Autodesk Inventor part; units mm, degrees
ref_plane "YZ Plane" through (0, 0, 0) normal (1, 0, 0) x (0, 1, 0)
ref_plane "XZ Plane" through (0, 0, 0) normal (0, 1, 0) x (-1, 0, 0)
ref_plane "XY Plane" through (0, 0, 0) normal (0, 0, 1) x (1, 0, 0)
sketch "Sketch1" plane through (0, 0, 0) normal (0, 1, 0) x (-1, 0, 0)
  line L0 (-25, 25) -> (-25, -25)
  line L1 (-25, -25) -> (25, -25)
  line L2 (25, -25) -> (25, 25)
  line L3 (25, 25) -> (-25, 25)
  line L4 (-25, 25) -> (25, -25) construction
  line L5 (-25, -25) -> (25, 25) construction
  point P0 (0, 0)
  dimension "d0" = 50
  dimension "d1" = 50
extrude "Extrusion1" add sketch "Sketch1" along normal blind 1
sketch "Sketch2" plane through (0, 1, 0) normal (0, 1, 0) x (1, 0, 0)
  line L0 (25, -25) -> (25, 25) construction
  line L1 (25, -25) -> (25, -20) construction
  line L2 (25, -20) -> (-25, -20) construction
  line L3 (-25, 25) -> (-25, -25) construction
  line L4 (25, -20) -> (25, -2) construction
  line L5 (25, -2) -> (-25, -2) construction
  line L6 (25, -20) -> (18, -20) construction
  line L7 (18, -20) -> (18, -2) construction
  line L8 (-25, -20) -> (-18, -20) construction
  line L9 (-18, -20) -> (-18, -2) construction
  line L10 (1, -2) -> (-1, -2) construction
  line L11 (-1, -2) -> (-1, -20) construction
  line L12 (-1, -20) -> (1, -20) construction
  line L13 (1, -20) -> (1, -2) construction
  line L14 (1, -2) -> (-1, -20) construction
  line L15 (-1, -2) -> (1, -20) construction
  line L16 (18, -2) -> (1, -2)
  line L17 (1, -2) -> (1, -20)
  line L18 (1, -20) -> (18, -20)
  line L19 (18, -20) -> (18, -2)
  line L20 (-1, -2) -> (-18, -2)
  line L21 (-18, -2) -> (-18, -20)
  line L22 (-18, -20) -> (-1, -20)
  line L23 (-1, -20) -> (-1, -2)
  point P0 (0, 0)
  point P1 (0, -11)
  dimension "d4" = 5
  dimension "d5" = 18
  dimension "d6" = 7
  dimension "d7" = 7
  dimension "d8" = 2
extrude "Extrusion2" add sketch "Sketch2" along normal blind 15
sketch "Sketch3" plane through (0, 1, 0) normal (0, 1, 0) x (1, 0, 0)
  line L0 (18, -20) -> (1, -20)
  line L1 (18, -20) -> (18, -25)
  line L2 (-25, -25) -> (25, -25)
  line L3 (1, -20) -> (1, -25)
  line L4 (1, -25) -> (18, -25)
  line L5 (18, -20) -> (1, -20)
  line L6 (18, -25) -> (12.33, -25)
  line L7 (12.33, -25) -> (12.33, -20)
  line L8 (18, -20) -> (12.33, -20)
  line L9 (12.33, -20) -> (6.66, -20)
  line L10 (6.66, -20) -> (6.66, -25)
  line L11 (6.66, -20) -> (1, -20)
  point P0 (0, 0)
  dimension "d11" = 5.67
  dimension "d12" = 5.67
extrude "Extrusion3" add sketch "Sketch3" along normal blind 11
sketch "Sketch4" plane through (18, 1, 25) normal (1, 0, 0) x (0, 0, -1)
  line L0 (5, 11) -> (5, 15)
  line L1 (5, 11) -> (4, 11)
  line L2 (0, 11) -> (5, 11)
  line L3 (4, 11) -> (5, 9.2085)
  line L4 (5, 0) -> (5, 15)
  point P0 (25, -1)
  dimension "d9" = 15
  dimension "d15" = 1
extrude "Extrusion4" cut sketch "Sketch4" against normal through all
sketch "Sketch5" plane through (0, 12, 0) normal (0, 1, 0) x (1, 0, 0)
  line L0 (18, -25) -> (18, -21) construction
  line L1 (18, -21) -> (12.33, -21) construction
  line L2 (18, -21) -> (1, -21) construction
  line L3 (12.33, -21) -> (12.33, -25.0141) construction
  line L4 (12.33, -25.0141) -> (6.66, -25) construction
  line L5 (1, -25) -> (18, -25) construction
  line L6 (6.66, -25) -> (6.67, -21) construction
  line L7 (6.67, -21) -> (1, -21) construction
  line L8 (-25, -25) -> (1, -25) construction
  line L9 (1, -21) -> (1, -25) construction
  circle A0 centre (3.835, -23) radius 1.625
  circle A1 centre (9.5, -23) radius 1.625
  circle A2 centre (15.165, -23) radius 1.625
  point P0 (0, 0)
  dimension "d18" = 5.67
  dimension "d19" = 5.67
  dimension "d20" = 5.67
  dimension "d21" = 3.25
  dimension "d22" = 3.25
  dimension "d23" = 3.25
extrude "Extrusion5" cut sketch "Sketch5" against normal blind 1.5
sketch "Sketch6" plane through (-25, 0, 25) normal (0, 0, 1) x (1, 0, 0)
  line L0 (0, 1) -> (26, 1)
  line L1 (26, 1) -> (43.0101, 1)
  line L2 (26, 12) -> (43, 12) construction
  line L3 (26, 12) -> (31.67, 12) construction
  line L4 (31.67, 12) -> (31.67, 1) construction
  line L5 (31.67, 1) -> (37.34, 1) construction
  line L6 (50, 1) -> (0, 1) construction
  line L7 (37.34, 1) -> (37.34, 12) construction
  line L8 (26.835, 6.1045) -> (30.835, 6.1045)
  line L9 (30.835, 6.1045) -> (30.835, 2.1045)
  line L10 (30.835, 2.1045) -> (26.835, 2.1045)
  line L11 (26.835, 2.1045) -> (26.835, 6.1045)
  line L12 (26.835, 6.1045) -> (30.835, 2.1045) construction
  line L13 (30.835, 6.1045) -> (26.835, 2.1045) construction
  point P0 (25, 0)
  point P1 (28.835, 4.1045)
  dimension "d26" = 5.67
  dimension "d27" = 5.67
  dimension "d28" = 4
  dimension "d29" = 4
extrude "Extrusion6" cut sketch "Sketch6" against normal blind 2
ref_plane "Work Plane1" through (9.5, 1, 2) normal (-1, 0, 0) x (0, 0, 1)
mirror "Mirror1" about plane through (9.5, 1, 2) normal (-1, 0, 0) of "Extrusion6"
ref_plane "Work Plane2" through (6.6675, 1, 2) normal (-1, 0, 0) x (0, 0, 1)
mirror "Mirror2" about plane through (6.6675, 1, 2) normal (-1, 0, 0) of "Extrusion6"
ref_plane "Work Plane3" through (0, 0, -25) normal (-1, 0, 0) x (0, 0, 1)
mirror "Mirror3" about plane through (0, 0, -25) normal (-1, 0, 0) of "Extrusion3", "Extrusion5", "Extrusion6", "Mirror1", "Mirror2", "Extrusion2"
sketch "Sketch7" plane through (0, 1, 0) normal (0, 1, 0) x (1, 0, 0)
  line L0 (25, 25) -> (25, 23) construction
  line L1 (25, -25) -> (25, 25) construction
  line L2 (25, 23) -> (23, 23) construction
  line L3 (23, 23) -> (13, 23)
  line L4 (13, 23) -> (13, 20.4297)
  line L5 (13, 20.4297) -> (23, 20.4297)
  line L6 (23, 20.4297) -> (23, 23)
  line L7 (18, 20.4297) -> (18, 23)
  line L8 (18, 20.4297) -> (23, 20.4297)
  line L9 (20.5, 20.4297) -> (20.5, 23)
  line L10 (18, 20.4297) -> (13, 20.4297)
  line L11 (15.5, 20.4297) -> (15.5, 23)
  circle A0 centre (21.75, 21.6797) radius 1.25
  circle A1 centre (19.25, 21.6797) radius 1.25
  circle A2 centre (16.75, 21.6797) radius 1.25
  circle A3 centre (14.25, 21.6797) radius 1.25
  circle A4 centre (21.75, 21.6797) radius 0.75
  circle A5 centre (19.25, 21.6797) radius 0.75
  circle A6 centre (16.75, 21.6797) radius 0.75
  circle A7 centre (14.25, 21.6797) radius 0.75
  point P0 (0, 0)
  dimension "d33" = 2
  dimension "d34" = 2
  dimension "d35" = 10
  dimension "d36" = 0.5
  dimension "d37" = 0.5
  dimension "d38" = 0.5
  dimension "d39" = 0.5
extrude "Extrusion7" add sketch "Sketch7" along normal blind 5 contours A4 | A5 | A6 | A7
extrude "Extrusion8" add sketch "Sketch7" along normal blind 1 contours L6 A0 L9 L3 | L9 A1 L7 L3 | A0 | L6 L5 A0 | L7 A2 L11 L3 | A0 L5 L9 | A1 | L9 L5 A1 | L11 A3 L4 L3 | A1 L5 L7 | A2 | L7 L5 A2 | A2 L5 L11 | A3 | L11 L5 A3 | A3 L5 L4 | A4 | A5 | A6 | A7
properties part number "H Bridge #2"
Here's how the part is built. I have some questions about the finished solid (model axes, mm). A direction names the side the tool comes from. Give positions to 0.01 mm unless a question says otherwise; leave off trailing zeros. Loops run counter-clockwise (first coordinate to the right, second up) from the corner with the lowest first, then second, coordinate; pieces in that order, holes last. Notation, with made-up numbers: M 72.25,25.25 L 95.25,25.25 A27 cw 95.25,55.25 Z; hole C 24,65 d9. An arc over 180 degrees is marked long. Return JSON: item names as keys, results as strings.
Item 1: Thinking about a two-plate mould opening in X: for faces 4 (the flat face through (-10, 14, 20)), 5 (the flat face through (9, 6.104, 24)), which applies, released by +X, released by -X, zero draft, split by the parting line, or undercut?
A:
{"face 4": "zero draft", "face 5": "undercut"}
Item 2: On a 3-axis mill with a long thin cutter (end or side, diameter ignored), from which of +Z, -Z, +X, -X, +Y, -Y can I reach the whole of each face in a straight line? I mean faces 1 (the flat face through (22, 6, -22)), 2 (the flat face through (-13.165, 4, 24)), 3 (the cylindrical face through (21, 3.97, -21.65)). Say none if no direction works.
A:
{"face 1": "+Z, -Z, +X, -X, +Y", "face 2": "+Z", "face 3": "+Y"}
Item 3: Imagine slicing it at A-A on y = 9. List the corners of the cut face in (x, z) for me.
A:
{"outline": "M -18,2 L -1,2 L -1,25 L -18,25 Z; M 1,2 L 18,2 L 18,25 L 1,25 Z"}
Item 4: I'm going to push flat-ended pins straight in: pin 1 Ø1.5 at (y, z) = (11.5, -0.5) entering from -X; pin 2 Ø0.6 at (y, z) = (4.5, 24) entering from +X; pin 3 Ø1.9 at (x, z) = (-3.835, 23) entering from +Y; pin 4 Ø3.5 at (x, z) = (3.835, 23) entering from +Y. Where does each tip first touch, or does it pass through?
A:
{"pin 1": "passes through", "pin 2": "stops at x = 18", "pin 3": "stops at y = 10.5", "pin 4": "stops at y = 12"}
Item 5: Imagine slicing it at C-C on z = 17. List the corners of the cut face in (x, y) for me.
A:
{"outline": "M -25,0 L 25,0 L 25,1 L 18,1 L 18,16 L 1,16 L 1,1 L -1,1 L -1,16 L -18,16 L -18,1 L -25,1 Z"}
Item 6: Please list where these lines run through material, in increasing order: line 1 (X direction, y = 14.75, z = 7.5); line 2 (Y direction, x = 19, z = -21.5); line 3 (Y direction, x = 8, z = -6).
A:
{"line 1": "x = -18 to -1, 1 to 18", "line 2": "y = 0 to 6", "line 3": "y = 0 to 1"}
